Drawing for the job (mm, zero at the part's lowest x, y, z). A direction names the side the tool comes from. Give positions to 0.01 mm unless a question says otherwise; leave off trailing zeros. Order: outer loops, then holes, each group sorted by start corner. A loop starts at its lowest first (then second) coordinate and runs counter-clockwise, first axis right, second up. Notation, with made-up numbers: (11, 31.25) - (22, 31.25) arc R10 ccw to (22, 47.25) - close; hole circle Ø2 at (12, -37). An arc over 180 degrees is marked (long way). Use CSV: the item, a comma, the result in double quotes. Start each with the question number.
(1) Band-saw the part on B-B, the plane x = 25.5. Give the cut face in (y, z).
(2) Band-saw the part on D-D, the plane z = 15. Give the cut face in (x, y).
(3) Tool access for the marked faces 1, 2, 3, 4 and 5: list every direction of +Z, -Z, +X, -X, +Y, -Y with a clear straight run to the whole face (end or side of a thin tool).
(4) Pull direction Z, two halves, no side cores. Call the marked faces 6, 7 and 8: +Z half, -Z half, draft (parallel to the pull), parting line (faces both ways), or undercut.
(5) Band-saw the part on A-A, the plane z = 9.5. Give the cut face in (x, y), then the cut area to 3 significant figures.
(6) Probe L1, parallel to Y at x = 27.5, z = 5; L2, parallel to X at y = 6.75, z = 9.5; L3, parallel to Y at x = 14.5, z = 5.5. List the from-to ranges inside material, lowest first.
(7) Drop a flat-ended pin along its axis: pin 1 Ø6.5 at (x, z) = (25.5, 9.5) entering from +Y. Give the stop position or say it passes through.
(8) Band-saw the part on C-C, the plane x = 43.5. Give the cut face in (y, z).
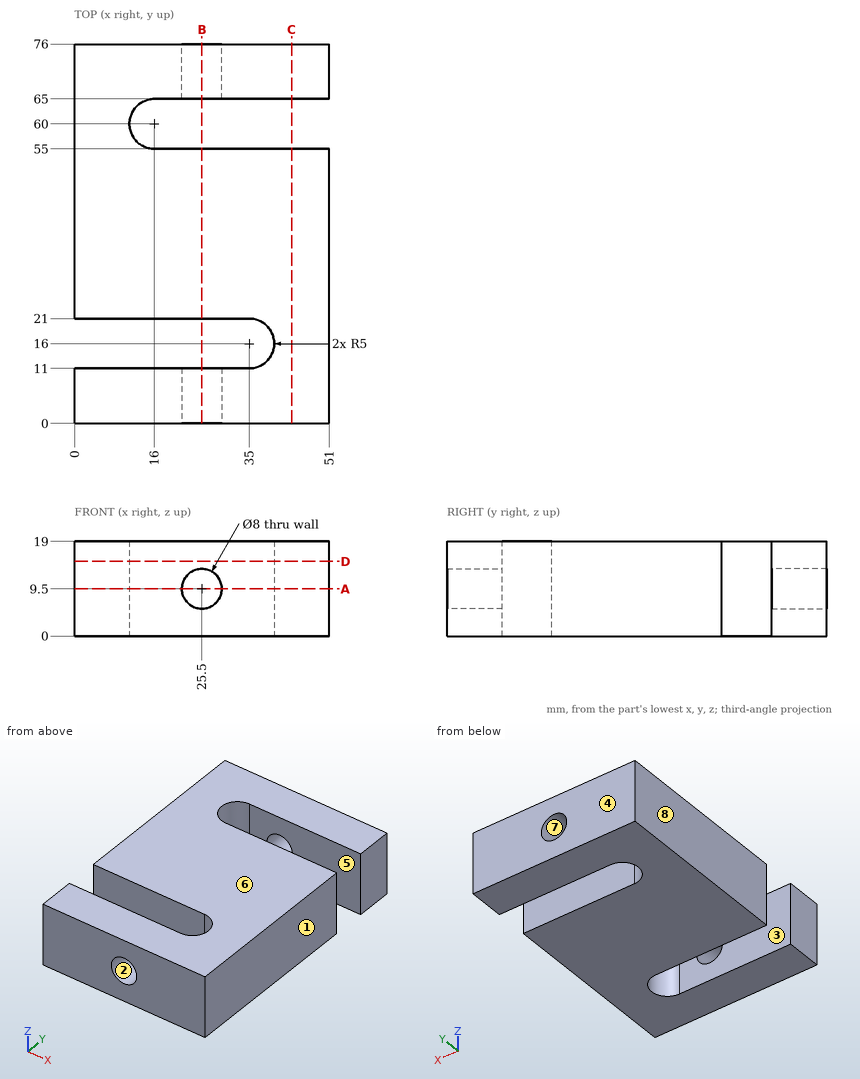
Answer block:
1,outline,"(0, 0) - (11, 0) - (11, 5.5) - (0, 5.5) - close; (0, 13.5) - (11, 13.5) - (11, 19) - (0, 19) - close; (21, 0) - (55, 0) - (55, 19) - (21, 19) - close; (65, 0) - (76, 0) - (76, 5.5) - (65, 5.5) - close; (65, 13.5) - (76, 13.5) - (76, 19) - (65, 19) - close"
2,outline,"(0, 0) - (51, 0) - (51, 55) - (16, 55) arc R5 cw to (16, 65) - (51, 65) - (51, 76) - (0, 76) - (0, 21) - (35, 21) arc R5 cw to (35, 11) - (0, 11) - close"
3,face 1,"+Z, -Z, +X, +Y, -Y"
3,face 2,"-Y"
3,face 3,"+Z, -Z, -X"
3,face 4,"+Z, -Z, +X, -X, +Y"
3,face 5,"+Z, -Z, +X"
4,face 6,"+Z half"
4,face 7,"undercut"
4,face 8,"draft"
5,outline,"(0, 0) - (21.5, 0) - (21.5, 11) - (0, 11) - close; (0, 21) - (35, 21) arc R5 cw to (35, 11) - (29.5, 11) - (29.5, 0) - (51, 0) - (51, 55) - (16, 55) arc R5 cw to (16, 65) - (21.5, 65) - (21.5, 76) - (0, 76) - close; (29.5, 65) - (51, 65) - (51, 76) - (29.5, 76) - close"
5,area,"2,920 mm2"
6,L1,"y = 0 to 11, 21 to 55, 65 to 76"
6,L2,"x = 0 to 21.5, 29.5 to 51"
6,L3,"y = 0 to 11, 21 to 55.23, 64.77 to 76"
7,pin 1,"stops at y = 55"
8,outline,"(0, 0) - (55, 0) - (55, 19) - (0, 19) - close; (65, 0) - (76, 0) - (76, 19) - (65, 19) - close"
